Autodesk Inventor part; units mm, degrees
ref_plane "YZ Plane" through (0, 0, 0) normal (1, 0, 0) x (0, 1, 0)
ref_plane "XZ Plane" through (0, 0, 0) normal (0, 1, 0) x (-1, 0, 0)
ref_plane "XY Plane" through (0, 0, 0) normal (0, 0, 1) x (1, 0, 0)
sketch "Sketch1" plane through (0, 0, 0) normal (0, 1, 0) x (-1, 0, 0)
  line L0 (0, 0) -> (111.2, 0)
  line L1 (116.2, 0) -> (116.2, -217)
  line L2 (116.2, -217) -> (0, -217)
  line L3 (0, -217) -> (0, 0)
  line L4 (111.2, 0) -> (111.2, 0)
  line L5 (111.2, 0) -> (116.2, 0)
  dimension "d4" = 5
  dimension "d5" = 111.2
  dimension "d6" = 217
  dimension "d7" = 217
extrude "Extrusion1" add sketch "Sketch1" along normal blind 5
fillet "Fillet1" radius 2 5 edges at (-111.2, 2.5, 0) (0, 2.5, 0) (-116.2, 2.5, 0) (0, 2.5, -217) (-116.2, 2.5, -217)
sketch "Sketch2" plane through (0, 5, 0) normal (0, 1, 0) x (1, 0, 0)
  line L0 (-12, -58.0921) -> (-12, 320.7627) construction
  line L1 (-43, -58.0921) -> (-43, 320.7627) construction
  line L2 (-149.1257, 202) -> (35.6079, 202) construction
  line L3 (-154.8253, 16) -> (27.8967, 16) construction
  line L4 (-114.2, 16) -> (-113.2, 16) construction
  line L5 (0, 2) -> (0, 215)
  point P0 (0, 0)
  point P1 (-43, 16)
  point P2 (-12, 16)
  point P3 (-43, 202)
  point P4 (-12, 202)
  dimension "d12" = 186
  dimension "d20" = 12
  dimension "d21" = 31
hole "Hole1" at (-43, 5, -16) at (-12, 5, -16) at (-43, 5, -202) at (-12, 5, -202) direction (0, -1, 0) diameter 4 end through all
properties part number "Central Divider"
Design review of the part built by this model. Coordinates are the model's own, in mm. Round coordinates to 2 decimals unless told otherwise and drop trailing zeros. Write each loop counter-clockwise with the first axis right and the second up, starting at its lowest first coordinate (ties: lowest second). Pieces come first, ordered by that corner, then holes. Notation, with made-up numbers: (-27.75, -1) - (6.25, -1) arc R17 cw to (6.25, 5) - close; hole circle Ø5 at (44, 28). An arc over 180 degrees is marked (long way). Use a Markdown table: item, result. Add a question column.
1. We need section A-A (x = -12). State the section outline as (y, z) points.
2. Mouldability with a two-part tool opening along X and no side actions: class faces 1 (the face through (-57, 2, 0)), 2 (the face through (-12, 2, -204)), 3 (the face through (0, 2, -110)) as +X half, -X half, draft (parallel to the pull), parting line (faces both ways), or undercut.
3. We need section B-B (z = -202). State the section outline as (x, y) points, then the cut area to 3 significant figures.
4. Wall thickness on probe 1 along X at (y, z) = (3.9, -202); probe 2 along Z at (x, y) = (-12, 1.55): over which ranges is each line inside the solid? List them lowest first.
Output:
| question | item | result |
|---|---|---|
| 1 | outline | (0, -217) - (5, -217) - (5, -204) - (0, -204) - close; (0, -200) - (5, -200) - (5, -18) - (0, -18) - close; (0, -14) - (5, -14) - (5, 0) - (0, 0) - close |
| 2 | face 1 | draft |
| 2 | face 2 | undercut |
| 2 | face 3 | +X half |
| 3 | outline | (-116.2, 0) - (-45, 0) - (-45, 5) - (-116.2, 5) - close; (-41, 0) - (-14, 0) - (-14, 5) - (-41, 5) - close; (-10, 0) - (0, 0) - (0, 5) - (-10, 5) - close |
| 3 | area | 541 mm2 |
| 4 | probe 1 | x = -116.2 to -45, -41 to -14, -10 to 0 |
| 4 | probe 2 | z = -217 to -204, -200 to -18, -14 to 0 |
